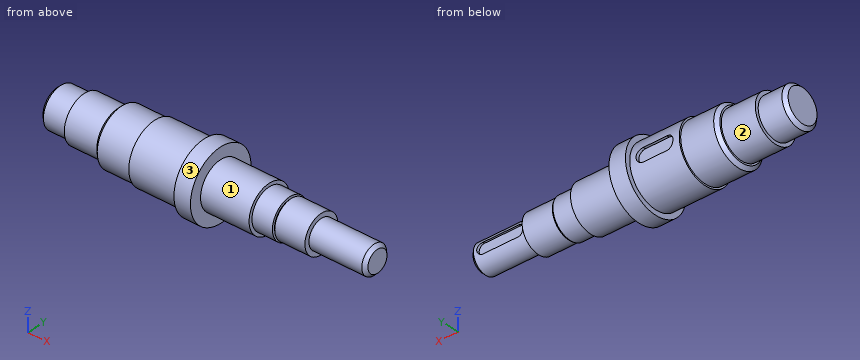
```python
from build123d import *

# Parameters (mm, degrees)
CHAMFER1_SIZE      = 5
CUT_EXTRUDE1_START = 45
CUT_EXTRUDE1_DEPTH = 4.9
CUT_EXTRUDE2_START = 21.5
CUT_EXTRUDE2_DEPTH = 4.3


with BuildPart() as part:
    # Sketch2 → Revolve1 (revolve)
    with BuildSketch(Plane(origin=(0, 0, 0), x_dir=(1, 0, 0), z_dir=(0, 1, 0)), mode=Mode.PRIVATE) as revolve1_sk:
        Polygon((242.5, 0), (-242.5, 0), (-242.5, 30), (-201.5, 30), (-201.5, 35), (-150, 35), (-150, 42.5), (-95, 42.5), (-95, 45), (-20, 45), (-20, 52.5), (5, 52.5), (5, 35), (78.55, 35), (78.55, 30), (109.55, 30), (109.55, 26.3), (111.75, 26.3), (111.75, 28.5), (157.5, 28.5), (157.5, 21.5), (242.5, 21.5), align=None)
    revolve(revolve1_sk.sketch.rotate(Axis((-418.822463349, 0, 0), (1, 0, 0)), 180), axis=Axis((-418.822463349, 0, 0), (1, 0, 0)))

    # Chamfer1
    chamfer1_edges = [part.edges().sort_by_distance(p)[0] for p in [
        (242.5, 0, -21.5),
        (-150, 0, -42.5),
        (-242.5, 0, -30),
    ]]
    chamfer(chamfer1_edges, length=CHAMFER1_SIZE)

    # Sketch3 → Cut-Extrude1 (cut, symmetric)
    with BuildSketch(Plane(origin=(0, 0, 0), x_dir=(1, 0, 0), z_dir=(0, 1, 0)).offset(CUT_EXTRUDE1_START)):
        with BuildLine():
            Line((-75.5, 10), (-39.5, 10))
            ThreePointArc((-39.5, 10), (-29.5, 0), (-39.5, -10))
            Line((-39.5, -10), (-75.5, -10))
            ThreePointArc((-75.5, -10), (-85.5, 0), (-75.5, 10))
        make_face()
    extrude(amount=CUT_EXTRUDE1_DEPTH, both=True, mode=Mode.SUBTRACT)

    # Sketch4 → Cut-Extrude2 (cut, symmetric)
    with BuildSketch(Plane(origin=(0, 0, 0), x_dir=(1, 0, 0), z_dir=(0, 1, 0)).offset(CUT_EXTRUDE2_START)):
        with BuildLine():
            Line((170.5, 8), (224.5, 8))
            ThreePointArc((224.5, 8), (232.5, 0), (224.5, -8))
            Line((224.5, -8), (170.5, -8))
            ThreePointArc((170.5, -8), (162.5, 0), (170.5, 8))
        make_face()
    extrude(amount=CUT_EXTRUDE2_DEPTH, both=True, mode=Mode.SUBTRACT)


solid = part.part
```
The listing builds one solid part. Answer for the finished solid, in the listing's coordinates (mm). Face numbers are marked on the shaded views. A direction names the side the tool comes from. Give positions to 0.01 mm unless a question says otherwise; leave off trailing zeros. Write each loop counter-clockwise with the first axis right and the second up, starting at its lowest first coordinate (ties: lowest second). Pieces come first, ordered by that corner, then holes. Notation, with made-up numbers: M -9,48.25 L 9,48.25 A8 ccw 9,61.25 Z; hole C 40.25,75 d2. An arc over 180 degrees is marked long. Write each question's results on one line, items separated by ' | '.
Q1. Section A-A, the plane x = -122 is taken. Write down the section's boundary in (y, z), then the cut area to 3 significant figures.
Output values:
outline: C 0,0 d85 | area: 5,670 mm2
Q2. Consider L1, parallel to X at y = -37, z = 35; L2, parallel to Z at x = -33, y = 40.5; L3, parallel to X at y = -10, z = 24.5. Determine where each line is inside the solid, lowest interval first. Write a range as from..to.
Output values:
L1: -20..5 | L2: -19.62..-7.6, 7.6..19.62 | L3: -241.04..109.55, 111.75..157.5
Q3. Section C-C, the plane x = 188 is taken. Write down the section's boundary in (y, z).
Output values:
outline: M 17.2,-8 L 17.2,8 L 19.96,8 A21.5 ccw long 19.96,-8 Z
Q4. A tool of negligible diameter and unlimited length cuts with its end or side. For the marked faces 1, 2 and 3, from which of +Z, -Z, +X, -X, +Y, -Y can it reach the whole face along a straight path? Write none if from no direction.
Output values:
face 1: +X | face 2: -X | face 3: +X, -X
Q5. Section B-B, the plane x = -211.5 is taken. Write down the section's boundary in (y, z), then the cut area to 3 significant figures.
Output values:
outline: C 0,0 d60 | area: 2,830 mm2
Q6. Flat-ended cylindrical pins translate along their axes: P1, Ø1.9, axis at x = -62, y = 42.5, coming from the -Z side; P2, Ø1.4, axis at x = 197.5, y = 18.5, coming from the -Z side; P3, Ø2, axis at x = 206.5, y = 18, coming from the +Z side. Find the tip coordinate at first contact, or state that the pin passes through.
Output values:
P1: z = -17.28 | P2: z = -12.06 | P3: z = 13.16
